The model under review builds one solid part; all positions refer to its coordinate system, in mm. Round coordinates to 2 decimals unless told otherwise and drop trailing zeros. Loops run counter-clockwise (first coordinate to the right, second up) from the corner with the lowest first, then second, coordinate; pieces in that order, holes last. Notation, with made-up numbers: M 43,38.5 L 87,38.5 A21 cw 87,47.5 Z; hole C 53.25,42 d11. An arc over 180 degrees is marked long. Return JSON: item names as keys, results as strings. Group by question number.
Q1. Consider section C-C (x = 36). State the section outline as (y, z) points, and give its area (3 significant figures).
Q2. Clearance check with a flat-ended pin moving along its axis: pin 1 Ø0.8 at (x, z) = (17.5, 0) entering from -Y. State where the tip first meets the part, or that it passes through.
Q3. Consider section A-A (z = 0.2). State the section outline as (x, y) points.
Q4. To check wall thickness, follow line 1 along Y through (x, z) = (14, -0.05); line 2 along X through (y, z) = (1.25, -0.1); line 3 along Y through (x, z) = (22.5, -0.35). State the ranges of each line that lie inside material, in increasing order.
Q5. Consider section D-D (x = 3.5). State the section outline as (y, z) points, and give its area (3 significant figures).
Q6. Consider section B-B (y = 4). State the section outline as (x, z) points.
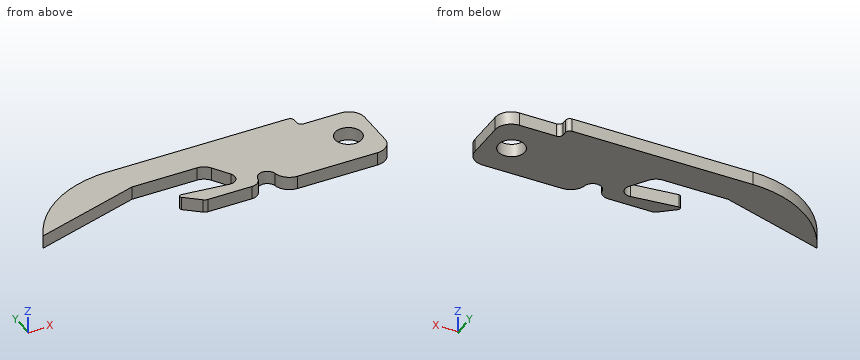
from build123d import *

# Parameters (mm, degrees)
SKETCH1_R           = 1.5
BOSS_EXTRUDE1_DEPTH = 0.75
FILLET1_R           = 1.8


with BuildPart() as part:
    # Sketch1 → Boss-Extrude1 (new, symmetric)
    with BuildSketch(Plane.XY):
        with BuildLine():
            Line((10.953994705, 9.5), (31.453994705, 9.5))
            ThreePointArc((31.453994705, 9.5), (31.807548096, 9.353553391), (31.953994705, 9))
            Line((31.953994705, 9), (31.953994705, 8.5))
            ThreePointArc((31.953994705, 8.5), (32.100441315, 8.146446609), (32.453994705, 8))
            Line((32.453994705, 8), (38.453994705, 8))
            Line((38.453994705, 8), (38.453994705, 0))
            Line((38.453994705, 0), (27.61132699, 0))
            ThreePointArc((27.61132699, 0), (26.453994705, 0.418752726), (25.83256534, 1.481107378))
            ThreePointArc((25.83256534, 1.481107378), (24.849102012, 2.3), (23.865638684, 1.481107378))
            ThreePointArc((23.865638684, 1.481107378), (23.453994705, 0.777387983), (22.687360725, 0.5))
            Line((22.687360725, 0.5), (17.705397605, 0.5))
            ThreePointArc((17.705397605, 0.5), (17.453994705, 0.543390786), (17.231681323, 0.668542449))
            Line((17.231681323, 0.668542449), (15.526396166, 2.057846521))
            ThreePointArc((15.526396166, 2.057846521), (15.453994705, 2.348921744), (15.713112665, 2.5))
            Line((15.713112665, 2.5), (20.884755714, 1.9))
            ThreePointArc((20.884755714, 1.9), (21.851554423, 2.369070966), (21.83503998, 3.44352645))
            Line((21.83503998, 3.44352645), (20.595191848, 5.325283904))
            ThreePointArc((20.595191848, 5.325283904), (20.053994705, 5.820591886), (19.342631878, 6))
            Line((19.342631878, 6), (11.953994705, 6))
            Line((11.953994705, 6), (0, 2.4))
            ThreePointArc((0, 2.4), (4.427127156, 7.5697567), (10.953994705, 9.5))
        make_face()
        with Locations((35.453994705, 4)):
            Circle(SKETCH1_R, mode=Mode.SUBTRACT)
    extrude(amount=BOSS_EXTRUDE1_DEPTH, both=True)

    # Fillet1
    fillet1_edges = [part.edges().sort_by_distance(p)[0] for p in [
        (38.453994705, 8, 0),
        (38.453994705, 0, 0),
    ]]
    fillet(fillet1_edges, radius=FILLET1_R)


solid = part.part
Values:
{
 "1": {"outline": "M 0,-0.75 L 2.6,-0.75 L 2.6,0.75 L 0,0.75 Z; M 5.4,-0.75 L 8,-0.75 L 8,0.75 L 5.4,0.75 Z", "area": "7.81 mm2"},
 "2": {"pin 1": "stops at y = 0.5"},
 "3": {"outline": "M 0,2.4 L 11.95,6 L 19.34,6 A1.5 cw 20.6,5.33 L 21.84,3.44 A1 cw 20.88,1.9 L 15.71,2.5 A0.25 ccw 15.53,2.06 L 17.23,0.67 A0.75 ccw 17.71,0.5 L 22.69,0.5 A1.2 ccw 23.87,1.48 A1 cw 25.83,1.48 A1.81 ccw 27.61,0 L 36.65,0 A1.8 ccw 38.45,1.8 L 38.45,6.2 A1.8 ccw 36.65,8 L 32.45,8 A0.5 cw 31.95,8.5 L 31.95,9 A0.5 ccw 31.45,9.5 L 10.95,9.5 A12 ccw Z; hole C 35.45,4 d3"},
 "4": {"line 1": "y = 6 to 9.5", "line 2": "x = 16.52 to 23.8, 25.89 to 38.37", "line 3": "y = 0.5 to 9.5"},
 "5": {"outline": "M 3.45,-0.75 L 6.9,-0.75 L 6.9,0.75 L 3.45,0.75 Z", "area": "5.18 mm2"},
 "6": {"outline": "M 0.87,-0.75 L 5.31,-0.75 L 5.31,0.75 L 0.87,0.75 Z; M 21.47,-0.75 L 33.95,-0.75 L 33.95,0.75 L 21.47,0.75 Z; M 36.95,-0.75 L 38.45,-0.75 L 38.45,0.75 L 36.95,0.75 Z"}
}
